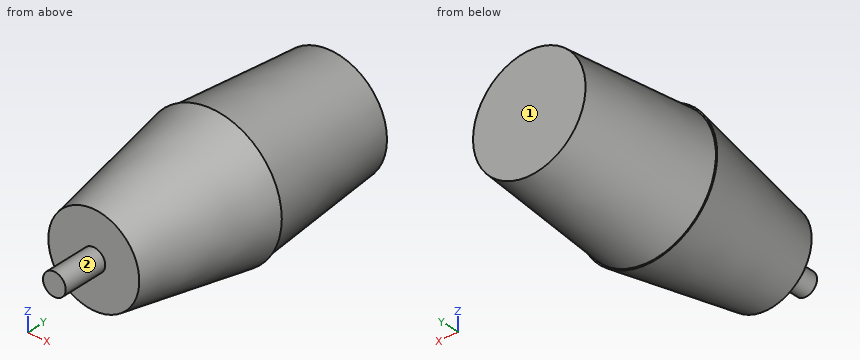
Autodesk Inventor part; units mm, degrees
ref_plane "YZ Plane" through (0, 0, 0) normal (1, 0, 0) x (0, 1, 0)
ref_plane "XZ Plane" through (0, 0, 0) normal (0, 1, 0) x (-1, 0, 0)
ref_plane "XY Plane" through (0, 0, 0) normal (0, 0, 1) x (1, 0, 0)
sketch "Sketch1" plane through (0, 0, 0) normal (0, 1, 0) x (-1, 0, 0)
  circle A0 centre (0, 0) radius 10
  dimension "d0" = 20
extrude "Extrusion1" add sketch "Sketch1" along normal blind 30 draft 10
sketch "Sketch2" plane through (0, 30, 0) normal (0, 1, 0) x (1, 0, 0)
  point P0 (0, 0)
sketch "Sketch3" plane through (0, 30, 0) normal (0, 1, 0) x (1, 0, 0)
  circle A0 centre (0, 0) radius 15
  dimension "d3" = 30
extrude "Extrusion2" add sketch "Sketch3" along normal blind 30 draft -5
sketch "Sketch4" plane through (0, 0, 0) normal (0, -1, 0) x (1, 0, 0)
  circle A0 centre (0, 0) radius 2.5
  dimension "d6" = 5
extrude "Extrusion3" add sketch "Sketch4" along normal blind 10
properties part number "torchHead"
The listing builds one solid part. Answer for the finished solid, in the listing's coordinates (mm). Face numbers are marked on the shaded views. A direction names the side the tool comes from. Coordinates: 2 decimals unless noted, no trailing zeros. Order: outer loops, then holes, each group sorted by start corner. A loop starts at its lowest first (then second) coordinate and runs counter-clockwise, first axis right, second up. Notation, with made-up numbers: M 5.25,-6.5 L 38.25,-6.5 A16 cw 38.25,3.5 Z; hole C 27.5,-22 d7. An arc over 180 degrees is marked long. Answer as a JSON object with one key per item and string values. Group by question number.
1. Section B-B on x = 0 is taken. Write down the section's boundary in (y, z).
2. Straight lines are drawn through the part: line 1 (Y direction, x = -7, z = -0.5); line 2 (Z direction, x = 9.5, y = 34.5); line 3 (Z direction, x = 4, y = 54.5). For each, find the intervals that lie inside material, in ascending order.
3. Section A-A on z = 0 is taken. Write down the section's boundary in (x, y).
4. A tool of negligible diameter and unlimited length cuts with its end or side. For the marked faces 1 and 2, from which of +Z, -Z, +X, -X, +Y, -Y can it reach the whole face along a straight path? Write none if from no direction.
5. Section D-D on y = 46 is taken. Write down the section's boundary in (x, z), then the cut area to 3 significant figures.
6. Flat-ended cylindrical pins translate along their axes: P1, Ø1, axis at y = 21, z = 8, coming from the -X side; P2, Ø2, axis at x = -10, y = 10.5, coming from the -Z side; P3, Ø10, axis at x = -8.5, y = 14.5, coming from the -Z side. Find the tip coordinate at first contact, or state that the pin passes through.
7. Section C-C on y = 14 is taken. Write down the section's boundary in (x, z).
Values follow:
{
 "1": {"outline": "M -10,-2.5 L 0,-2.5 L 0,-10 L 30,-15.29 L 30,-15 L 60,-12.38 L 60,12.38 L 30,15 L 30,15.29 L 0,10 L 0,2.5 L -10,2.5 Z"},
 "2": {"line 1": "0 to 60", "line 2": "-11.09 to 11.09", "line 3": "-12.22 to 12.22"},
 "3": {"outline": "M -15.29,30 L -10,0 L -2.5,0 L -2.5,-10 L 2.5,-10 L 2.5,0 L 10,0 L 15.29,30 L 15,30 L 12.38,60 L -12.38,60 L -15,30 Z"},
 "4": {"face 1": "+Z, -Z, +X, -X, +Y", "face 2": "-Y"},
 "5": {"outline": "C 0,0 d27.2", "area": "581 mm2"},
 "6": {"P1": "x = -11.48", "P2": "z = -7.74", "P3": "z = -12.31"},
 "7": {"outline": "C 0,0 d24.94"}
}
